The model under review builds one solid part; all positions refer to its coordinate system, in mm. A direction names the side the tool comes from. Round coordinates to 2 decimals unless told otherwise and drop trailing zeros. Write each loop counter-clockwise with the first axis right and the second up, starting at its lowest first coordinate (ties: lowest second). Pieces come first, ordered by that corner, then holes. Notation, with made-up numbers: (-36, 89.25) -> (11, 89.25) arc R21 cw to (11, 118.25) -> close; hole circle Ø5 at (-13, 51.25). An arc over 180 degrees is marked (long way). Return JSON: item names as keys, results as strings. Group by question number.
1. Clearance check with a flat-ended pin moving along its axis: P1, Ø3, axis at x = -25.4, z = 12.7, coming from the +Y side. State where the tip first meets the part, or that it passes through.
2. Tool access review of faces 4 (the flat face through (-1.524, 13, 221)), 5 (the flat face through (-27, 1, 447.675)): name each direction out of +Z, -Z, +X, -X, +Y, -Y from which nothing blocks a thin tool from reaching the whole face with its end or side.
3. Take a section at A-A, the plane x = -6. Write out the cut boundary in (y, z) (3 decimals).
4. Take a section at B-B, the plane y = 19. Write out the cut boundary in (x, z) (3 decimals), then the cut area to 3 significant figures.
5. Mouldability with a two-part tool opening along Y and no side actions: class faces 1 (the flat face through (-26, 1.524, 221)), 2 (the flat face through (-26, 0, 221)), 3 (the flat face through (-50.8, 13, 221)) as pulls with the +Y half, pulls with the -Y half, needs draft (parallel to the pull), parting line crosses it, or undercut.
6. For line 1 along X through (y, z) = (25, 12.7); line 2 along Y through (x, z) = (-20, 129); line 3 along X through (y, z) = (20.5, 72), list the stretches that pass through material, from the lowest coordinate up. Write a range as from..to.
7. Take a section at C-C, the plane z = 409.5. Write out the cut boundary in (x, y).
from build123d import *

# Parameters (mm, degrees)
SKETCH1_W               = 50.8
SKETCH1_H               = 25.4
SKETCH1_W_2             = 47.752
SKETCH1_H_2             = 22.352
EXTRUDE_THIN1_DEPTH     = 447.675
CUT_EXTRUDE1_DEPTH      = 452.263454786
CUT_EXTRUDE1_DEPTH_BACK = 452.263454786
SKETCH2_R               = 2.38125


with BuildPart() as part:
    # Sketch1 → Extrude-Thin1 (new body)
    with BuildSketch(Plane.XY):
        with Locations((-25.4, 12.7)):
            Rectangle(SKETCH1_W, SKETCH1_H)
        with Locations((-25.4, 12.7)):
            Rectangle(SKETCH1_W_2, SKETCH1_H_2, mode=Mode.SUBTRACT)
    extrude(amount=EXTRUDE_THIN1_DEPTH)

    # Sketch2 → Cut-Extrude1 (cut, two sides: drawn at the far end of the back side and taken through both)
    with BuildSketch(Plane(origin=(0, 25.4, 0), x_dir=(1, 0, 0), z_dir=(0, 1, 0)).offset(-CUT_EXTRUDE1_DEPTH_BACK)):
        with Locations(Location((-38.1, -434.975, 0), (0, 0, 180))):
            Circle(SKETCH2_R)
        with Locations(Location((-25.4, -434.975, 0), (0, 0, 180))):
            Circle(SKETCH2_R)
        with Locations(Location((-12.7, -434.975, 0), (0, 0, 180))):
            Circle(SKETCH2_R)
        with Locations(Location((-38.1, -12.7, 0), (0, 0, 90))):
            Circle(SKETCH2_R)
        with Locations(Location((-12.7, -12.7, 0), (0, 0, 90))):
            Circle(SKETCH2_R)
        with Locations(Location((-25.4, -12.7, 0), (0, 0, 90))):
            Circle(SKETCH2_R)
    extrude(amount=CUT_EXTRUDE1_DEPTH + CUT_EXTRUDE1_DEPTH_BACK, mode=Mode.SUBTRACT)


solid = part.part
Output:
{
 "1": {"P1": "passes through"},
 "2": {"face 4": "+Z, -Z", "face 5": "+Z, +X, -X, +Y, -Y"},
 "3": {"outline": "(0, 0) -> (1.524, 0) -> (1.524, 447.675) -> (0, 447.675) -> close; (23.876, 0) -> (25.4, 0) -> (25.4, 447.675) -> (23.876, 447.675) -> close"},
 "4": {"outline": "(-50.8, 0) -> (-49.276, 0) -> (-49.276, 447.675) -> (-50.8, 447.675) -> close; (-1.524, 0) -> (0, 0) -> (0, 447.675) -> (-1.524, 447.675) -> close", "area": "1,360 mm^2"},
 "5": {"face 1": "undercut", "face 2": "pulls with the -Y half", "face 3": "needs draft"},
 "6": {"line 1": "x = -50.8..-40.48, -35.72..-27.78, -23.02..-15.08, -10.32..0", "line 2": "y = 0..1.52, 23.88..25.4", "line 3": "x = -50.8..-49.28, -1.52..0"},
 "7": {"outline": "(-50.8, 0) -> (0, 0) -> (0, 25.4) -> (-50.8, 25.4) -> close; hole (-49.28, 1.52) -> (-1.52, 1.52) -> (-1.52, 23.88) -> (-49.28, 23.88) -> close"}
}
